Part model, mm, in its own coordinate system. A direction names the side the tool comes from. Coordinates: 2 decimals unless noted, no trailing zeros. Write each loop counter-clockwise with the first axis right and the second up, starting at its lowest first coordinate (ties: lowest second). Pieces come first, ordered by that corner, then holes. Notation, with made-up numbers: (3.5, -26) - (43.5, -26) arc R18 ccw to (43.5, 2) - close; hole circle Ø6 at (86.25, 67.25). An arc over 180 degrees is marked (long way). Use a Markdown table: item, result.
Autodesk Inventor part; units mm, degrees
ref_plane "YZ Plane" through (0, 0, 0) normal (1, 0, 0) x (0, 1, 0)
ref_plane "XZ Plane" through (0, 0, 0) normal (0, 1, 0) x (-1, 0, 0)
ref_plane "XY Plane" through (0, 0, 0) normal (0, 0, 1) x (1, 0, 0)
sketch "Sketch1" plane through (0, 0, 0) normal (0, 0, 1) x (1, 0, 0)
  line L0 (0, 0) -> (25.4, 0)
  line L1 (25.4, 0) -> (25.4, 25.4)
  line L2 (25.4, 25.4) -> (0, 25.4)
  line L3 (0, 25.4) -> (0, 0)
  line L4 (3.175, 22.225) -> (22.225, 22.225)
  line L5 (22.225, 22.225) -> (22.225, 3.175)
  line L6 (22.225, 3.175) -> (3.175, 3.175)
  line L7 (3.175, 3.175) -> (3.175, 22.225)
  dimension "d0" = 25.4
  dimension "d1" = 25.4
  dimension "d2" = 3.175
extrude "Extrusion1" add sketch "Sketch1" along normal blind 609.6
sketch "Sketch2" plane through (0, 25.4, 0) normal (0, 1, 0) x (1, 0, 0)
  line L0 (25.4, 0) -> (25.4, -609.6)
  line L1 (25.4, -609.6) -> (0, -609.6)
  point P0 (0, 0)
  point P1 (12.7, -596.9)
  dimension "d12" = 12.7
  dimension "d13" = 12.7
hole "Hole1" at (12.7, 25.4, 596.9) direction (0, -1, 0) diameter 6.35 end through all
sketch "Sketch3" plane through (0, 25.4, 0) normal (0, 1, 0) x (1, 0, 0)
  line L0 (25.4, 0) -> (0, 0)
  line L1 (25.4, 0) -> (25.4, -609.6)
  point P0 (12.7, -12.7)
  dimension "d14" = 12.7
  dimension "d15" = 12.7
hole "Hole2" at (12.7, 25.4, 12.7) direction (0, -1, 0) diameter 6.35 end through all
pattern_linear "Rectangular Pattern1" count 2 spacing 25.4 along (0, 0, -1) count 2 spacing 25.4 along (0, 0, 1) of "Hole1", "Hole2"
sketch "Sketch4" plane through (25.4, 0, 0) normal (1, 0, 0) x (0, 0, -1)
  line L0 (0, 25.4) -> (-609.6, 25.4)
  line L1 (-609.6, 0) -> (-609.6, 25.4)
  line L2 (0, 0) -> (0, 25.4)
  point P0 (-596.9, 12.7)
  point P1 (-12.7, 12.7)
  dimension "d29" = 12.7
  dimension "d30" = 12.7
  dimension "d31" = 12.7
  dimension "d32" = 12.7
hole "Hole3" at (25.4, 12.7, 596.9) at (25.4, 12.7, 12.7) direction (-1, 0, 0) diameter 5.08 end through all
pattern_linear "Rectangular Pattern2" count 2 spacing 25.4 along (0, 0, -1) count 2 spacing 25.4 along (0, 0, 1) of "Hole3"
sketch "Sketch5" plane through (0, 25.4, 0) normal (0, 1, 0) x (1, 0, 0)
  line L0 (25.4, 0) -> (25.4, -609.6)
  circle A0 centre (12.7, -571.5) radius 3.175
  point P0 (0, 0)
  point P1 (12.7, -533.4)
  dimension "d46" = 12.7
  dimension "d54" = 38.1
hole "Hole4" at (12.7, 25.4, 533.4) direction (0, -1, 0) diameter 6.35 end through all
pattern_linear "Rectangular Pattern3" count 10 spacing 50.8 along (0, 0, -1) of "Hole4"
sketch "Sketch6" plane through (25.4, 0, 0) normal (1, 0, 0) x (0, 0, -1)
  line L0 (0, 25.4) -> (-609.6, 25.4)
  line L1 (-609.6, 0) -> (-609.6, 25.4)
  point P0 (0, 0)
  point P1 (-495.3, 12.7)
  dimension "d58" = 12.7
  dimension "d66" = 114.3
hole "Hole5" at (25.4, 12.7, 495.3) direction (-1, 0, 0) diameter 6.35 end through all
pattern_linear "Rectangular Pattern4" count 4 spacing 127 along (0, 0, -1) of "Hole5"
equation "\"d0\" = d1"
properties part number "testRoboRescue_Chassis_Frame_widthBar" material "Aluminum 6061"
Item 1: Drill centre lines: probe 1 along Y at (x, z) = (5.5, 359.5) (3 decimals); probe 2 along Y at (x, z) = (2.3, 368.3) (3 decimals). Where is each one in solid material? Low to high.
From the geometry:
| item | result |
|---|---|
| probe 1 | 0 to 3.175, 22.225 to 25.4 |
| probe 2 | 0 to 9.525, 15.875 to 25.4 |
Item 2: Band-saw the part on A-A, the plane z = 265. Give the cut face in (x, y) (3 decimals), then the cut area to 3 significant figures.
From the geometry:
| item | result |
|---|---|
| outline | (0, 0) - (25.4, 0) - (25.4, 25.4) - (0, 25.4) - close; hole (3.175, 3.175) - (22.225, 3.175) - (22.225, 22.225) - (3.175, 22.225) - close |
| area | 282 mm^2 |
Item 3: Two-plate mould, pull along X, no slides. Class faces 3 (the face through (13, 0, 301)), 4 (the face through (13, 22.225, 301)), 5 (the face through (25.4, 13, 301)), 6 (the face through (13, 3.175, 301)): pulls with the +X half, pulls with the -X half, needs draft (parallel to the pull), parting line crosses it, or undercut.
From the geometry:
| item | result |
|---|---|
| face 3 | needs draft |
| face 4 | undercut |
| face 5 | pulls with the +X half |
| face 6 | undercut |
Item 4: Which spindle directions (+Z, -Z, +X, -X, +Y, -Y) get a long thin tool onto all of the face, cutting with end or side? Do faces 1 (the face through (22.225, 13, 301)), 2 (the face through (13, 25.4, 301)). Say none if no direction does.
From the geometry:
| item | result |
|---|---|
| face 1 | +Z, -Z |
| face 2 | +Z, -Z, +X, -X, +Y |
